Source: three-view drawing plus pictorial views. Frame: mm from the lowest corner of the part. A direction names the side the tool comes from. Coordinates: 2 decimals unless noted, no trailing zeros. Write each loop counter-clockwise with the first axis right and the second up, starting at its lowest first coordinate (ties: lowest second). Pieces come first, ordered by that corner, then holes. Notation, with made-up numbers: M -23.5,-14.75 L 27.5,-14.75 A13 ccw 27.5,6.25 Z; hole C 41,45.25 d11. An arc over 180 degrees is marked long. Use CSV: the item, a comma, the result in double quotes.
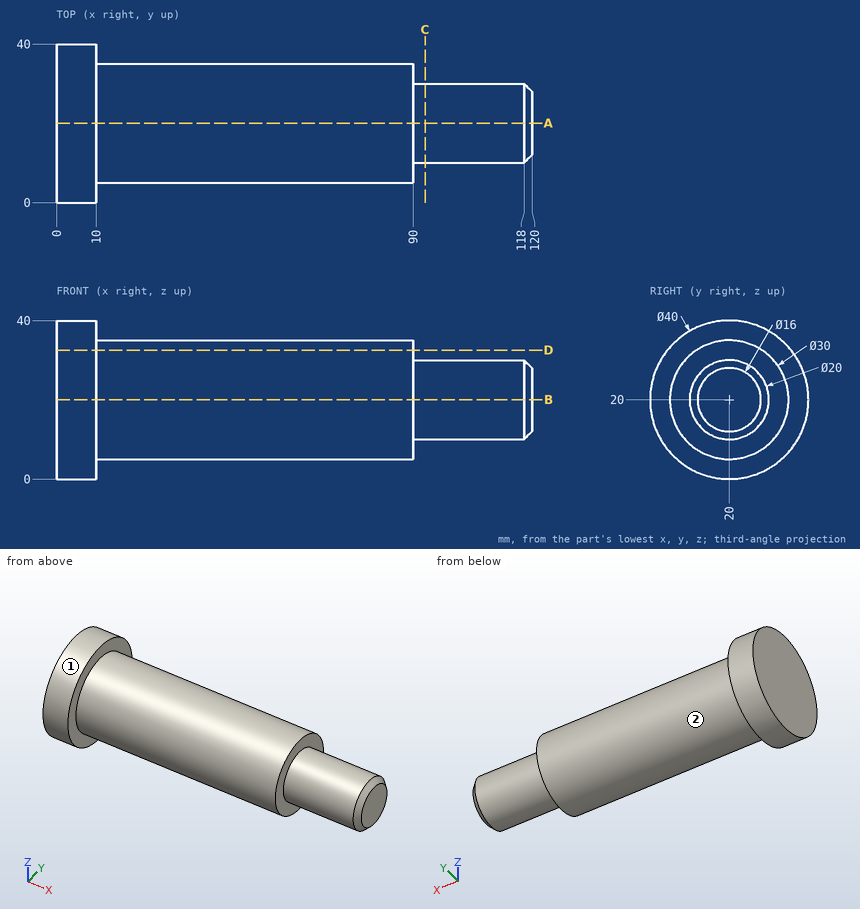
1. Section C-C (x = 93). Return loops of the section in (y, z).
Resolved:
outline,"C 20,20 d20"
2. Contact query for flat-ended pins moving along their axis: pin 1 Ø1 at (x, y) = (38, 27) entering from +Z; pin 2 Ø3 at (x, z) = (83, 10) entering from +Y; pin 3 Ø6 at (x, y) = (27.5, 19) entering from +Z. Output: stop coordinate, or through.
Resolved:
pin 1,"stops at z = 33.52"
pin 2,"stops at y = 32.36"
pin 3,"stops at z = 35"
3. Section A-A (y = 20). Return loops of the section in (x, z).
Resolved:
outline,"M 0,0 L 10,0 L 10,5 L 90,5 L 90,10 L 118,10 L 120,12 L 120,28 L 118,30 L 90,30 L 90,35 L 10,35 L 10,40 L 0,40 Z"
4. Material intervals for line 1 (X direction, y = 34.5, z = 23.5); line 2 (X direction, y = 8.5, z = 4.5); line 3 (Z direction, x = 13, y = 23.5), sorted ascending. Write a range as [from, to].
Resolved:
line 1,"x = [0, 90]"
line 2,"x = [0, 10]"
line 3,"z = [5.41, 34.59]"
5. Section D-D (z = 32.5). Return loops of the section in (x, y), then the cut area to 3 significant figures.
Resolved:
outline,"M 0,4.39 L 10,4.39 L 10,11.71 L 90,11.71 L 90,28.29 L 10,28.29 L 10,35.61 L 0,35.61 Z"
area,"1,640 mm^2"
6. Access query for the marked faces 1 and 2. Directions: +Z, -Z, +X, -X, +Y, -Y. A direction counts if a zero-diameter tool reaches every point of the face in a straight line with its end or side. Return the directions, or none.
Resolved:
face 1,"+X, -X"
face 2,"+X"
